Verification items for the finished model (mm, model axes). Face numbers are marked on the shaded views. A direction names the side the tool comes from. Round coordinates to 2 decimals unless told otherwise and drop trailing zeros. Order: outer loops, then holes, each group sorted by start corner. A loop starts at its lowest first (then second) coordinate and runs counter-clockwise, first axis right, second up. Notation, with made-up numbers: (0, 23) -> (10, 23) arc R15 ccw to (10, 33) -> close; hole circle Ø11 at (-37.75, -24). An arc over 180 degrees is marked (long way). Return JSON: item names as keys, results as strings. Group by question number.
Item 1: Scan lines: probe 1 along X at (y, z) = (10, 0); probe 2 along Z at (x, y) = (18.5, 18.5); probe 3 along X at (y, z) = (15.5, -1.25). Record each from-to range of solid material in increasing order. Write a range as from..to.
Item 2: Depth check by flat-ended pin: pin 1 Ø4 at (x, z) = (5.5, -5.5) entering from +Y; pin 2 Ø4 at (x, y) = (-4.5, 7.5) entering from -Z; pin 3 Ø7.5 at (x, y) = (21.5, 8) entering from -Z; pin 4 Ø2.5 at (x, z) = (-15, 0) entering from +Y. Enter the tip coordinate at first touch or a pass-through.
Item 3: Sectioned sample at A-A on x = 15. Record the cut outline in (y, z).
Item 4: Access from +Z, -Z, +X, -X, +Y, -Y to the whole of each face (thin tool, end or side, straight path). Record for the marked faces 1, 2, 3, 4 and 5.
Item 5: Draft check along Z on the marked faces 6, 7, 8 and 9. Enter one of: pulls with the +Z half, pulls with the -Z half, needs draft (parallel to the pull), parting line crosses it, or undercut.
Item 6: Sectioned sample at D-D on z = 0. Record the cut outline in (x, y), plus the area to 4 significant figures.
Item 7: Sectioned sample at B-B on y = 23.5. Record the cut outline in (x, z), plus the area to 3 significant figures.
Item 8: Sectioned sample at C-C on y = 2.75. Record the cut outline in (x, z).
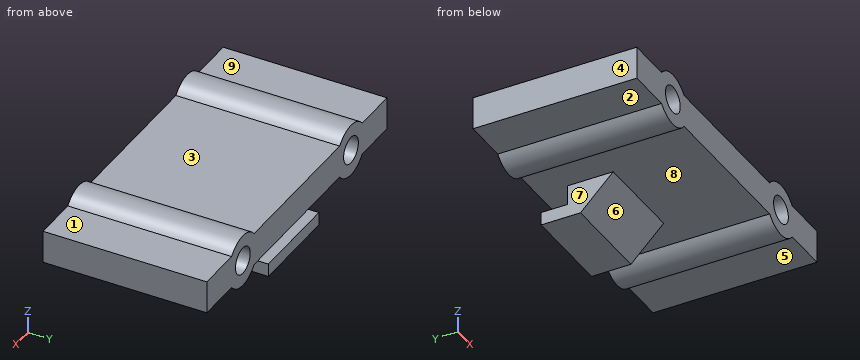
```python
from build123d import *

# Parameters (mm, degrees)
SKETCH1_R           = 2.05
BOSS_EXTRUDE1_DEPTH = 25
SKETCH2_W           = 14
SKETCH2_H           = 2
BOSS_EXTRUDE2_DEPTH = 5
SKETCH3_W           = 14
SKETCH3_H           = 2
BOSS_EXTRUDE3_DEPTH = 4
RIB3_REACH          = 43.295
SKETCH4_WALL_W      = 91.660413372
SKETCH4_WALL_H      = 14


with BuildPart() as part:
    # Sketch1 → Boss-Extrude1 (new body)
    with BuildSketch(Plane(origin=(0, 0, 0), x_dir=(1, 0, 0), z_dir=(0, 1, 0))):
        with BuildLine():
            Line((-25, 2.5), (-18.122498999, 2.5))
            ThreePointArc((-18.122498999, 2.5), (-15, 4), (-11.877501001, 2.5))
            Line((-11.877501001, 2.5), (11.877501001, 2.5))
            ThreePointArc((11.877501001, 2.5), (15, 4), (18.122498999, 2.5))
            Line((18.122498999, 2.5), (25, 2.5))
            Line((25, 2.5), (25, -2.5))
            Line((25, -2.5), (18.122498999, -2.5))
            ThreePointArc((18.122498999, -2.5), (15, -4), (11.877501001, -2.5))
            Line((11.877501001, -2.5), (-11.877501001, -2.5))
            ThreePointArc((-11.877501001, -2.5), (-15, -4), (-18.122498999, -2.5))
            Line((-18.122498999, -2.5), (-25, -2.5))
            Line((-25, -2.5), (-25, 2.5))
        make_face()
        with Locations(Location((-15, 0, 0), (0, 0, 270))):
            Circle(SKETCH1_R, mode=Mode.SUBTRACT)
        with Locations(Location((15, 0, 0), (0, 0, 270))):
            Circle(SKETCH1_R, mode=Mode.SUBTRACT)
    extrude(amount=BOSS_EXTRUDE1_DEPTH)

    # Sketch2 → Boss-Extrude2 (add)
    with BuildSketch(Plane(origin=(0, 0, -2.5), x_dir=(-1, 0, 0), z_dir=(0, 0, -1))):
        with Locations((0, 19.5)):
            Rectangle(SKETCH2_W, SKETCH2_H)
    extrude(amount=BOSS_EXTRUDE2_DEPTH)

    # Sketch3 → Boss-Extrude3 (add)
    with BuildSketch(Plane(origin=(0, 20.5, 0), x_dir=(1, 0, 0), z_dir=(0, 1, 0))):
        with Locations((0, 6.5)):
            Rectangle(SKETCH3_W, SKETCH3_H)
    extrude(amount=BOSS_EXTRUDE3_DEPTH)

    # Sketch4 wall → Rib3 (add, up to next)
    with BuildSketch(Plane(origin=(-7, 16, -5), x_dir=(0, -0.707106781187, 0.707106781187), z_dir=(0, 0.707106781187, 0.707106781187)), mode=Mode.PRIVATE) as rib3_sk1:
        with Locations((0, 7)):
            Rectangle(SKETCH4_WALL_W, SKETCH4_WALL_H)
    rib3_tool1 = extrude(rib3_sk1.sketch, amount=RIB3_REACH, mode=Mode.PRIVATE) - part.part
    add(rib3_tool1.solids().sort_by_distance((-7, 16, -5))[0])


solid = part.part
```
Recorded:
{
 "1": {"probe 1": "-25..-17.05, -12.95..12.95, 17.05..25", "probe 2": "-2.5..2.5", "probe 3": "-25..-16.62, -13.38..13.38, 16.62..25"},
 "2": {"pin 1": "y = 24.5", "pin 2": "z = -2.5", "pin 3": "z = -2.9", "pin 4": "through"},
 "3": {"outline": "(0, -4) -> (25, -4) -> (25, -2.05) -> (0, -2.05) -> close; (0, 2.05) -> (25, 2.05) -> (25, 4) -> (0, 4) -> close"},
 "4": {"face 1": "+Z, +X, +Y, -Y", "face 2": "-Z, -X, +Y, -Y", "face 3": "+Z, +Y, -Y", "face 4": "+Z, -Z, -X, +Y, -Y", "face 5": "-Z, +X, +Y, -Y"},
 "5": {"face 6": "pulls with the -Z half", "face 7": "needs draft", "face 8": "undercut", "face 9": "pulls with the +Z half"},
 "6": {"outline": "(-25, 0) -> (-17.05, 0) -> (-17.05, 25) -> (-25, 25) -> close; (-12.95, 0) -> (12.95, 0) -> (12.95, 25) -> (-12.95, 25) -> close; (17.05, 0) -> (25, 0) -> (25, 25) -> (17.05, 25) -> close", "area": "1,045 mm²"},
 "7": {"outline": "(-25, -2.5) -> (-18.12, -2.5) arc R4 ccw to (-11.88, -2.5) -> (11.88, -2.5) arc R4 ccw to (18.12, -2.5) -> (25, -2.5) -> (25, 2.5) -> (18.12, 2.5) arc R4 ccw to (11.88, 2.5) -> (-11.88, 2.5) arc R4 ccw to (-18.12, 2.5) -> (-25, 2.5) -> close; (-7, -7.5) -> (7, -7.5) -> (7, -5.5) -> (-7, -5.5) -> close; hole circle Ø4.1 at (-15, 0); hole circle Ø4.1 at (15, 0)", "area": "278 mm²"},
 "8": {"outline": "(-25, -2.5) -> (-18.12, -2.5) arc R4 ccw to (-11.88, -2.5) -> (11.88, -2.5) arc R4 ccw to (18.12, -2.5) -> (25, -2.5) -> (25, 2.5) -> (18.12, 2.5) arc R4 ccw to (11.88, 2.5) -> (-11.88, 2.5) arc R4 ccw to (-18.12, 2.5) -> (-25, 2.5) -> close; hole circle Ø4.1 at (-15, 0); hole circle Ø4.1 at (15, 0)"}
}
